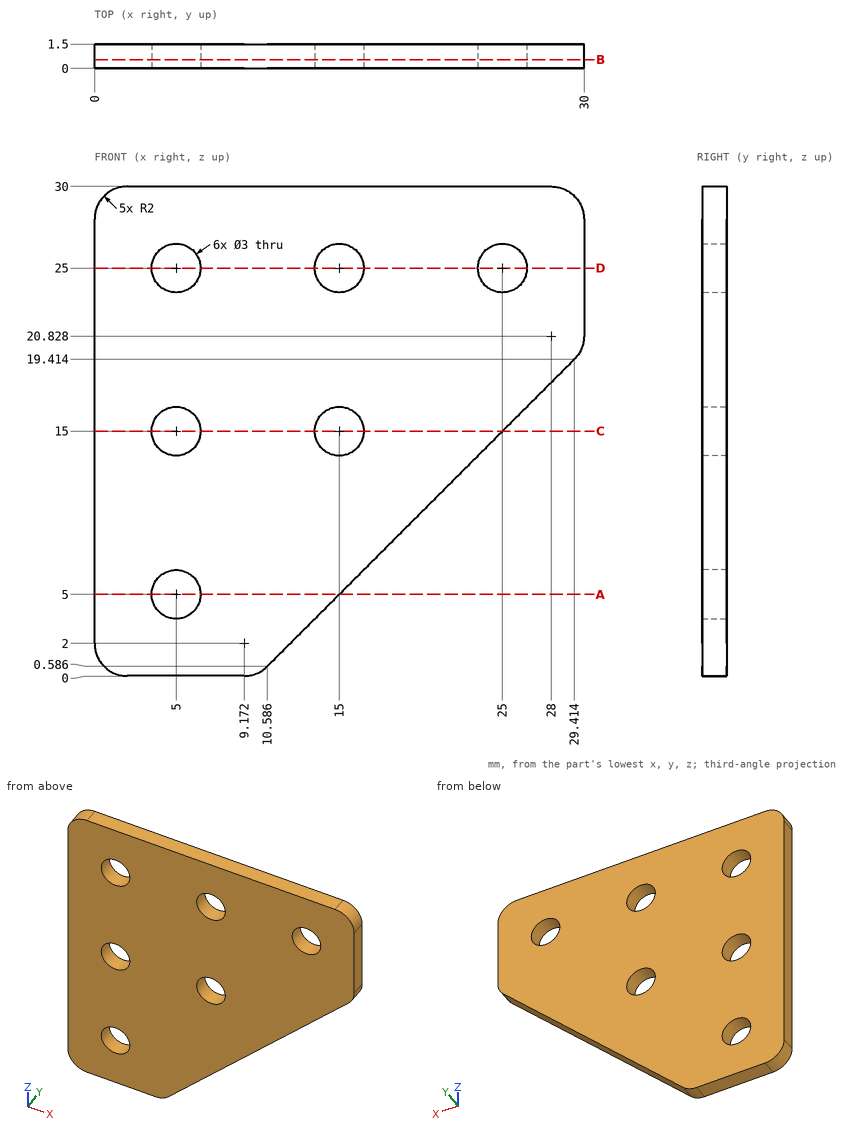
Can you work these out from the drawing? Everything is in mm from the part's minimum corner. Round coordinates to 2 decimals unless told otherwise and drop trailing zeros. Order: outer loops, then holes, each group sorted by start corner. A loop starts at its lowest first (then second) coordinate and runs counter-clockwise, first axis right, second up. Notation, with made-up numbers: M 72,24.5 L 94,24.5 A30 ccw 94,60.5 Z; hole C -4,-14.75 d6. An arc over 180 degrees is marked long. One line per question, with ' | ' between items.
1) I need wall thicknesses on line 1 along X through (y, z) = (0.65, 25); line 2 along Z through (x, y) = (3.75, 1.25); line 3 along X through (y, z) = (0.8, 15). Which ranges of each line are inside material? Lowest first, please.
Working result:
line 1: 0 to 3.5, 6.5 to 13.5, 16.5 to 23.5, 26.5 to 30 | line 2: 0 to 4.17, 5.83 to 14.17, 15.83 to 24.17, 25.83 to 30 | line 3: 0 to 3.5, 6.5 to 13.5, 16.5 to 25
2) For pin 1 Ø1.8 at (x, z) = (15, 25) entering from +Y, with a flat end and sliding along its axis, tell me the tip position at first contact or that it passes through.
Working result:
pin 1: through
3) I want a section at C-C, the plane z = 15. Write out the boundary of the cut face in (x, y).
Working result:
outline: M 0,0 L 3.5,0 L 3.5,1.5 L 0,1.5 Z; M 6.5,0 L 13.5,0 L 13.5,1.5 L 6.5,1.5 Z; M 16.5,0 L 25,0 L 25,1.5 L 16.5,1.5 Z
4) I want a section at B-B, the plane y = 0.55. Write out the boundary of the cut face in (x, z) (1 decimal).
Working result:
outline: M 0,2 A2 ccw 2,0 L 9.2,0 A2 ccw 10.6,0.6 L 29.4,19.4 A2 ccw 30,20.8 L 30,28 A2 ccw 28,30 L 2,30 A2 ccw 0,28 Z; hole C 5,5 d3; hole C 5,15 d3; hole C 5,25 d3; hole C 15,15 d3; hole C 15,25 d3; hole C 25,25 d3
5) I want a section at A-A, the plane z = 5. Write out the boundary of the cut face in (x, y), then the cut area to 3 significant figures.
Working result:
outline: M 0,0 L 3.5,0 L 3.5,1.5 L 0,1.5 Z; M 6.5,0 L 15,0 L 15,1.5 L 6.5,1.5 Z | area: 18.0 mm²
6) I want a section at D-D, the plane z = 25. Write out the boundary of the cut face in (x, y).
Working result:
outline: M 0,0 L 3.5,0 L 3.5,1.5 L 0,1.5 Z; M 6.5,0 L 13.5,0 L 13.5,1.5 L 6.5,1.5 Z; M 16.5,0 L 23.5,0 L 23.5,1.5 L 16.5,1.5 Z; M 26.5,0 L 30,0 L 30,1.5 L 26.5,1.5 Z
